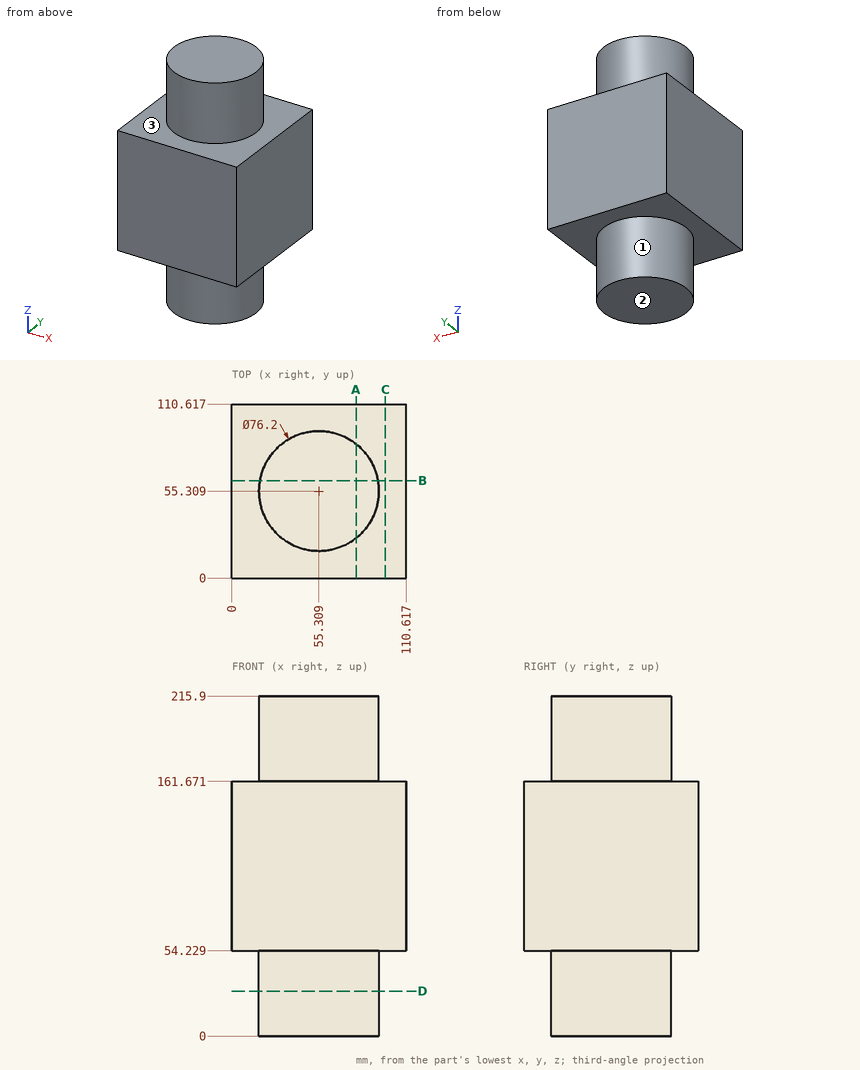
For this review, use the dimensioned drawing (mm, ordinates from the lowest corner) and the shaded views. A direction names the side the tool comes from. Coordinates: 2 decimals unless noted, no trailing zeros. Order: outer loops, then holes, each group sorted by start corner. A loop starts at its lowest first (then second) coordinate and runs counter-clockwise, first axis right, second up. Notation, with made-up numbers: M -13.5,87.5 L 44.5,87.5 A13 cw 44.5,108.5 Z; hole C 22,6.25 d6. An arc over 180 degrees is marked long. Answer as a JSON object with one key per item and string values. Group by question number.
1) Add section A-A, the plane x = 79. Write out the cut boundary in (y, z), then the cut area to 3 significant figures.
2) Add section B-B, the plane y = 62. Write out the cut boundary in (x, z), then the cut area to 3 significant figures.
3) For pin 1 (12 mm diameter, centred on x = 45, z = 37.5, fed in from +Y); pin 2 (1.5 mm diameter, centred on x = 37.5, z = 52, fed in from +Y), all flat-tipped, find the tip position at first contact; note any pin that passes through.
4) Add section D-D, the plane z = 28.5. Write out the cut boundary in (x, y).
5) Wall thickness on L1, parallel to Z at x = 17, y = 30; L2, parallel to X at y = 55.5, z = 174.5; L3, parallel to Y at x = 62, z = 44 (1 decimal): over which ranges is each line inside the solid? List them lowest first.
6) Tool access review of the marked faces 1, 2 and 3: name each direction out of +Z, -Z, +X, -X, +Y, -Y from which nothing blocks a thin tool from reaching the whole face with its end or side.
7) Add section C-C, the plane x = 97.5. Write out the cut boundary in (y, z).
Computed values:
{
 "1": {"outline": "M 0,54.23 L 25.47,54.23 L 25.47,0 L 85.15,0 L 85.15,54.23 L 110.62,54.23 L 110.62,161.67 L 85.15,161.67 L 85.15,215.9 L 25.47,215.9 L 25.47,161.67 L 0,161.67 Z", "area": "18,400 mm^2"},
 "2": {"outline": "M 0,54.23 L 17.8,54.23 L 17.8,0 L 92.82,0 L 92.82,54.23 L 110.62,54.23 L 110.62,161.67 L 92.82,161.67 L 92.82,215.9 L 17.8,215.9 L 17.8,161.67 L 0,161.67 Z", "area": "20,000 mm^2"},
 "3": {"pin 1": "stops at y = 93.16", "pin 2": "stops at y = 89.38"},
 "4": {"outline": "C 55.31,55.31 d76.2"},
 "5": {"L1": "z = 54.23 to 161.67", "L2": "x = 17.21 to 93.41", "L3": "y = 17.8 to 92.8"},
 "6": {"face 1": "-Z", "face 2": "-Z, +X, -X, +Y, -Y", "face 3": "+Z"},
 "7": {"outline": "M 0,54.23 L 110.62,54.23 L 110.62,161.67 L 0,161.67 Z"}
}
